from build123d import *

# Parameters (mm, degrees)
F0_W     = 350
F0_H     = 195
F1_DEPTH = 10
F3_D     = 6
F5_D     = 3.5
F5_DEPTH = 5
F5_TIP   = 1.0515060833


with BuildPart() as f1:
    # F0 (on Top) → F1 (new body, symmetric)
    with BuildSketch(Plane.XY):
        Rectangle(F0_W, F0_H)
    extrude(amount=F1_DEPTH, both=True)

    # F3 (through all)
    with Locations(Plane.XZ.offset(97.5)):
        with Locations((-125, 0), (-75, 0), (75, 0), (125, 0)):
            Hole(F3_D / 2)

    # F5
    with Locations(Plane(origin=(0, 0, -10), x_dir=(1, 0, 0), z_dir=(0, 0, -1))):
        with Locations((-49, 5), (-49, -5), (-39, 0), (65, 5), (65, -5), (75, 0)):
            Hole(F5_D / 2, depth=F5_DEPTH)
            with Locations((0, 0, -(F5_DEPTH + F5_TIP / 2))):  # 118° drill point
                Cone(0, F5_D / 2, F5_TIP, mode=Mode.SUBTRACT)


solid = f1.part
Can you work these out from the model? Positions are in its coordinate system, mm. Coordinates: 2 decimals unless noted, no trailing zeros. Loops run counter-clockwise (first coordinate to the right, second up) from the corner with the lowest first, then second, coordinate; pieces in that order, holes last. Notation, with made-up numbers: M 8,54.5 L 49,54.5 A27 cw 49,79.5 Z; hole C -23,-40 d2. An arc over 180 degrees is marked long. Return JSON: item names as keys, results as strings. Group by question number.
Item 1: If I drill on L1, parallel to X at y = -5, z = -6.5; L2, parallel to Y at x = -49, z = -8.7; L3, parallel to Y at x = 75, z = -6.65, over which ranges is the centre line in solid material (lowest first)? Write a range as from..to.
Item 2: Imagine slicing it at B-B (y = -59). Please give me the cut outline in (x, z).
Item 3: I'm going to push flat-ended pins straight in: pin 1 Ø3.5 at (x, z) = (75, 0) entering from +Y; pin 2 Ø5.5 at (x, y) = (65, -5) entering from -Z; pin 3 Ø2 at (x, y) = (75, 0) entering from -Z; pin 4 Ø3 at (x, y) = (-49, 5) entering from -Z. Where does each tip first touch, or does it pass through?
Item 4: Imagine slicing it at A-A (z = 0). Please give me the cut outline in (x, y).
Verdict:
{
 "1": {"L1": "x = -175..-50.75, -47.25..63.25, 66.75..175", "L2": "y = -97.5..-6.75, -3.25..3.25, 6.75..97.5", "L3": "y = -97.5..-1.75, 1.75..97.5"},
 "2": {"outline": "M -175,-10 L 175,-10 L 175,10 L -175,10 Z; hole C -125,0 d6; hole C -75,0 d6; hole C 75,0 d6; hole C 125,0 d6"},
 "3": {"pin 1": "passes through", "pin 2": "stops at z = -10", "pin 3": "stops at z = -4.55", "pin 4": "stops at z = -4.85"},
 "4": {"outline": "M -175,-97.5 L -128,-97.5 L -128,97.5 L -175,97.5 Z; M -122,-97.5 L -78,-97.5 L -78,97.5 L -122,97.5 Z; M -72,-97.5 L 72,-97.5 L 72,97.5 L -72,97.5 Z; M 78,-97.5 L 122,-97.5 L 122,97.5 L 78,97.5 Z; M 128,-97.5 L 175,-97.5 L 175,97.5 L 128,97.5 Z"}
}
